Part model, mm, in its own coordinate system. Round coordinates to 2 decimals unless told otherwise and drop trailing zeros. Write each loop counter-clockwise with the first axis right and the second up, starting at its lowest first coordinate (ties: lowest second). Pieces come first, ordered by that corner, then holes. Notation, with made-up numbers: (42, 36.5) -> (65, 36.5) arc R10 ccw to (65, 50.5) -> close; hole circle Ø1 at (86, 75.5). An arc over 180 degrees is marked (long way). Use CSV: the item, a comma, the result in double quotes. Start each with the question number.
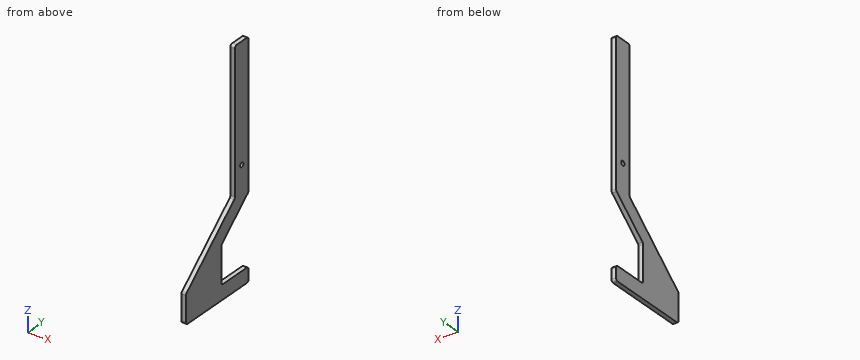
```python
from build123d import *

# Parameters (mm, degrees)
SKETCH1_R           = 1.5
BOSS_EXTRUDE1_DEPTH = 1.5
FILLET1_R           = 1.5875


with BuildPart() as part:
    # Sketch1 → Boss-Extrude1 (new, symmetric)
    with BuildSketch(Plane(origin=(0, 0, 0), x_dir=(0, 0, -1), z_dir=(1, 0, 0))):
        Polygon((-75.668068816, 16.486293283), (-75.668068816, 29.186293283), (20.071657388, 29.186293283), (41.38478802, 3.786293283), (66.143068816, 3.786293283), (66.143068816, 29.186293283), (75.668068816, 29.186293283), (75.668068816, -29.186293283), (56.618068816, -29.186293283), (18.294218273, 16.486293283), align=None)
        with Locations((0.531931184, 22.836293283)):
            Circle(SKETCH1_R, mode=Mode.SUBTRACT)
    extrude(amount=BOSS_EXTRUDE1_DEPTH, both=True)

    # Fillet1
    fillet1_edges = [part.edges().sort_by_distance(p)[0] for p in [
        (0, 29.186293283, -20.071657388),
        (0, 3.786293283, -41.38478802),
        (0, 3.786293283, -66.143068816),
        (0, 29.186293283, -66.143068816),
        (0, 29.186293283, -75.668068816),
        (0, -29.186293283, -75.668068816),
        (0, -29.186293283, -56.618068816),
        (0, 16.486293283, -18.294218273),
        (0, 16.486293283, 75.668068816),
        (0, 29.186293283, 75.668068816),
    ]]
    fillet(fillet1_edges, radius=FILLET1_R)


solid = part.part
```
1. Band-saw the part on C-C (z = -13.5). List the corners of the cut face in (x, y).
2. Drill centre lines: line 1 along Z through (x, y) = (-0.8, 19); line 2 along Y through (x, z) = (-0.7, 54); line 3 along Z through (x, y) = (-1.25, 6). Where is each one in solid material? Low to high. Write a range as [from, to].
3. Band-saw the part on A-A (x = 0.05). List the corners of the cut face in (y, z) (1 decimal), then the cut area to 3 significant figures.
4. Band-saw the part on B-B (y = -11.5). List the corners of the cut face in (x, z).
Answers below:
1,outline,"(-1.5, 16.49) -> (1.5, 16.49) -> (1.5, 29.19) -> (-1.5, 29.19) -> close"
2,line 1,"z = [-75.67, -66.14], [-28.62, 75.67]"
2,line 2,"y = [16.49, 29.19]"
2,line 3,"z = [-75.67, -66.14], [-39.53, -27.09]"
3,outline,"(-29.2, -74.1) arc R1.6 ccw to (-27.6, -75.7) -> (27.6, -75.7) arc R1.6 ccw to (29.2, -74.1) -> (29.2, -67.7) arc R1.6 ccw to (27.6, -66.1) -> (5.4, -66.1) arc R1.6 cw to (3.8, -64.6) -> (3.8, -42.1) arc R1.6 cw to (4.4, -40.9) -> (28.6, -20.5) arc R1.6 ccw to (29.2, -19.3) -> (29.2, 74.1) arc R1.6 ccw to (27.6, 75.7) -> (18.1, 75.7) arc R1.6 ccw to (16.5, 74.1) -> (16.5, -17.6) arc R1.6 cw to (15.9, -18.8) -> (-28.6, -56.1) arc R1.6 ccw to (-29.2, -57.4) -> close; hole circle Ø3 at (22.8, -0.5)"
3,area,"2,760 mm^2"
4,outline,"(-1.5, -75.67) -> (1.5, -75.67) -> (1.5, -41.78) -> (-1.5, -41.78) -> close"
